Build history of the part. All positions in model axes, mm. Give positions to 0.01 mm unless a question says otherwise; leave off trailing zeros. Order: outer loops, then holes, each group sorted by start corner. A loop starts at its lowest first (then second) coordinate and runs counter-clockwise, first axis right, second up. Notation, with made-up numbers: (83.25, -1) - (119.25, -1) arc R24 cw to (119.25, 13) - close; hole circle Ø1 at (73.5, -8). An arc over 180 degrees is marked (long way). Answer in a Markdown table with one row per item.
```python
from build123d import *

# Parameters (mm, degrees)
SKETCH1_W           = 57.15
SKETCH1_H           = 57.15
SKETCH1_R           = 25.4
SKETCH1_R_2         = 2.15265
SKETCH1_R_3         = 3.99923
BOSS_EXTRUDE1_DEPTH = 6.35
SKETCH1_3_W         = 57.15
SKETCH1_3_H         = 57.15
SKETCH1_3_R         = 25.4
SKETCH1_3_R_2       = 2.15265
BOSS_EXTRUDE2_DEPTH = 38.1
FILLET1_R           = 3
CHAMFER1_SIZE       = 0.3


with BuildPart() as part:
    # Sketch1 → Boss-Extrude1 (new body)
    with BuildSketch(Plane.XY):
        Rectangle(SKETCH1_W, SKETCH1_H)
        Circle(SKETCH1_R, mode=Mode.SUBTRACT)
        with Locations((-23.622, -23.622)):
            Circle(SKETCH1_R_2, mode=Mode.SUBTRACT)
        with Locations((23.622, -23.622)):
            Circle(SKETCH1_R_2, mode=Mode.SUBTRACT)
        with Locations((23.622, 23.622)):
            Circle(SKETCH1_R_2, mode=Mode.SUBTRACT)
        with Locations((-23.622, 23.622)):
            Circle(SKETCH1_R_2, mode=Mode.SUBTRACT)
        Circle(SKETCH1_R)
        Circle(SKETCH1_R_3, mode=Mode.SUBTRACT)
    extrude(amount=BOSS_EXTRUDE1_DEPTH)

    # Sketch1_3 → Boss-Extrude2 (add)
    with BuildSketch(Plane.XY):
        Rectangle(SKETCH1_3_W, SKETCH1_3_H)
        with Locations(Location((0, 0, 0), (0, 0, 180))):
            Circle(SKETCH1_3_R, mode=Mode.SUBTRACT)
        with Locations((-23.622, -23.622)):
            Circle(SKETCH1_3_R_2, mode=Mode.SUBTRACT)
        with Locations((23.622, -23.622)):
            Circle(SKETCH1_3_R_2, mode=Mode.SUBTRACT)
        with Locations((23.622, 23.622)):
            Circle(SKETCH1_3_R_2, mode=Mode.SUBTRACT)
        with Locations((-23.622, 23.622)):
            Circle(SKETCH1_3_R_2, mode=Mode.SUBTRACT)
    extrude(amount=BOSS_EXTRUDE2_DEPTH)

    # Fillet1
    fillet1_edges = [part.edges().sort_by_distance(p)[0] for p in [
        (28.575, 28.575, 19.05),
        (28.575, -28.575, 19.05),
        (-28.575, -28.575, 19.05),
        (-28.575, 28.575, 19.05),
    ]]
    fillet(fillet1_edges, radius=FILLET1_R)

    # Chamfer1
    chamfer1_edges = [part.edges().sort_by_distance(p)[0] for p in [
        (-3.99923, 0, 6.35),
        (-25.77465, 23.622, 0),
        (21.46935, 23.622, 0),
        (21.46935, -23.622, 0),
        (-25.77465, -23.622, 0),
        (-3.99923, 0, 0),
        (-25.77465, 23.622, 38.1),
        (21.46935, 23.622, 38.1),
        (21.46935, -23.622, 38.1),
        (-25.77465, -23.622, 38.1),
        (25.4, 0, 38.1),
        (-28.575, 0, 0),
        (-28.575, 0, 38.1),
        (0, 28.575, 0),
        (28.575, 0, 0),
        (0, -28.575, 0),
        (-27.696320344, -27.696320344, 0),
        (27.696320344, -27.696320344, 0),
        (27.696320344, 27.696320344, 0),
        (-27.696320344, 27.696320344, 0),
        (0, 28.575, 38.1),
        (0, -28.575, 38.1),
        (28.575, 0, 38.1),
        (-27.696320344, -27.696320344, 38.1),
        (27.696320344, -27.696320344, 38.1),
        (27.696320344, 27.696320344, 38.1),
        (-27.696320344, 27.696320344, 38.1),
    ]]
    chamfer(chamfer1_edges, length=CHAMFER1_SIZE)


solid = part.part
```
1. Cut at C-C on z = 12.5. Write the cut outline in (x, y) (3 decimals).
Check result:
| item | result |
|---|---|
| outline | (-28.575, -25.575) arc R3 ccw to (-25.575, -28.575) - (25.575, -28.575) arc R3 ccw to (28.575, -25.575) - (28.575, 25.575) arc R3 ccw to (25.575, 28.575) - (-25.575, 28.575) arc R3 ccw to (-28.575, 25.575) - close; hole circle Ø4.305 at (-23.622, -23.622); hole circle Ø4.305 at (-23.622, 23.622); hole circle Ø50.8 at (0, 0); hole circle Ø4.305 at (23.622, -23.622); hole circle Ø4.305 at (23.622, 23.622) |
2. Probe line 1 (Y direction, x = 0, z = 3.85) (3 decimals); line 2 (Y direction, x = 22.5, z = 2) (3 decimals); line 3 (Y direction, x = 0, z = 18) (3 decimals). List the from-to ranges inside material, lowest first.
Check result:
| item | result |
|---|---|
| line 1 | y = -28.575 to -3.999, 3.999 to 28.575 |
| line 2 | y = -28.575 to -25.459, -21.785 to 21.785, 25.459 to 28.575 |
| line 3 | y = -28.575 to -25.4, 25.4 to 28.575 |
3. Cut at A-A on y = 0. Write the cut outline in (x, z) (3 decimals), and give its area (3 significant figures).
Check result:
| item | result |
|---|---|
| outline | (-28.575, 0.3) - (-28.275, 0) - (-4.299, 0) - (-3.999, 0.3) - (-3.999, 6.05) - (-4.299, 6.35) - (-25.4, 6.35) - (-25.4, 37.8) - (-25.7, 38.1) - (-28.275, 38.1) - (-28.575, 37.8) - close; (3.999, 0.3) - (4.299, 0) - (28.275, 0) - (28.575, 0.3) - (28.575, 37.8) - (28.275, 38.1) - (25.7, 38.1) - (25.4, 37.8) - (25.4, 6.35) - (4.299, 6.35) - (3.999, 6.05) - close |
| area | 513 mm² |
4. Two-plate mould, pull along Y, no slides. Class faces 1 (the face through (21.914, 22.312, 18.788)), 2 (the face through (0, 7, 0)), 3 (the face through (-0.867, -3.904, 3.135)), 4 (the face through (27.72, -27.67, 19.31)): +Y half, -Y half, draft (parallel to the pull), parting line (faces both ways), or undercut.
Check result:
| item | result |
|---|---|
| face 1 | undercut |
| face 2 | draft |
| face 3 | undercut |
| face 4 | -Y half |
5. Cut at D-D on x = -23. Count the separate pieces of the cut face and the enclosed holes in it, and give its area (3 significant figures).
Check result:
| item | result |
|---|---|
| separate pieces | 3 |
| enclosed holes | 0 |
| area | 1,180 mm² |
6. Drop a flat-ended pin along its axis: P1, Ø5, axis at x = -19.5, y = -8.5, coming from the +Z side. Give the stop position or say it passes through.
Check result:
| item | result |
|---|---|
| P1 | stops at z = 6.35 |
